Could you check a few things on this drawing? It's one solid part, dimensions in mm from its lowest x, y, z. A direction names the side the tool comes from. Coordinates: 2 decimals unless noted, no trailing zeros. Use one line per item in the form item = value. Start each with the question number.
(1) On a 3-axis mill with a long thin cutter (end or side, diameter ignored), from which of +Z, -Z, +X, -X, +Y, -Y can I reach the whole of each face in a straight line? I mean the marked faces 3 and 4. Say none if no direction works.
(2) Thinking about a two-plate mould opening in X: for the marked faces 1 and 2, which applies, +X half, -X half, draft (parallel to the pull), parting line (faces both ways), or undercut?
(3) Please list where these lines run through material, in increasing order: L1, parallel to Y at x = 20.5, z = 30; L2, parallel to Z at x = 31.5, y = 1.55; L3, parallel to X at y = 0.8, z = 53.5 (1 decimal).
(4) Will these pins go through, and if not, where does the flat tip stop? P1, Ø2, axis at x = 48, y = 2, coming from the -Z side; P2, Ø1, axis at y = 4, z = 37.5, coming from the +X side; P3, Ø3, axis at y = 1.5, z = 8, coming from the +X side (1 decimal).
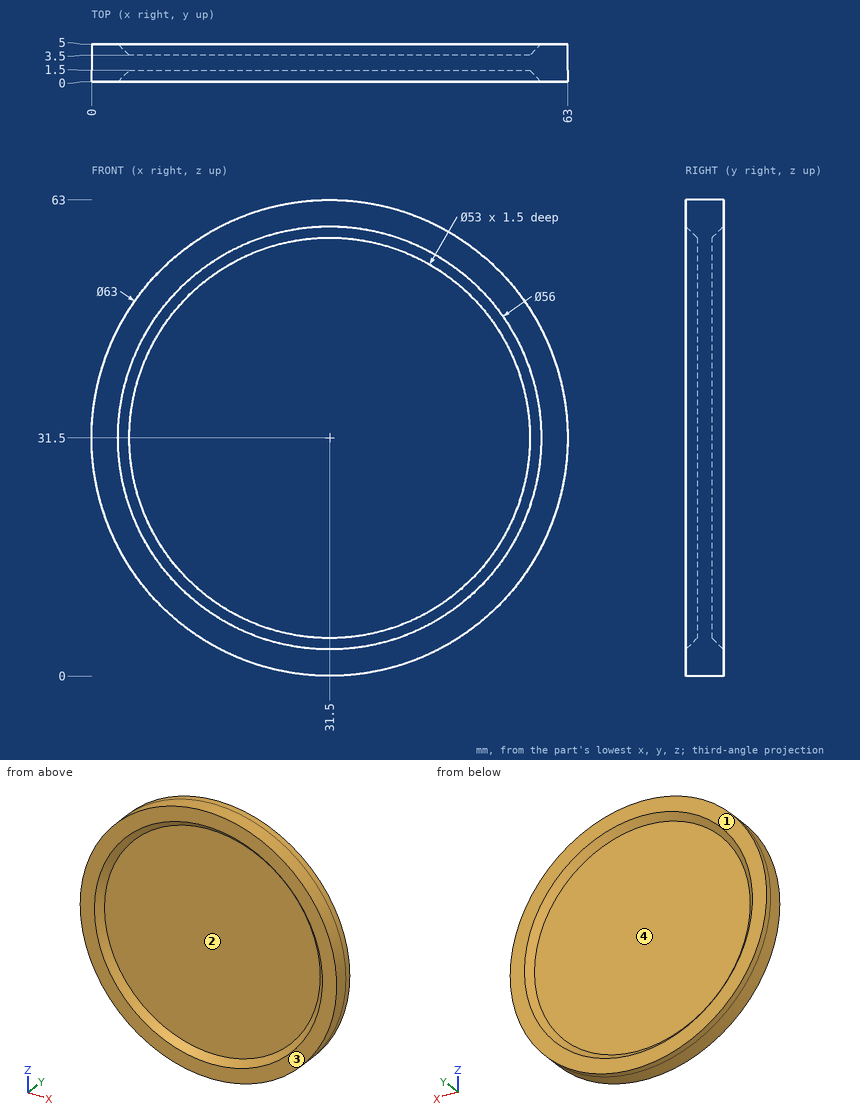
Answer:
q1.face_3 = +Z, -Z, +X, -X, -Y
q1.face_4 = +Y
q2.face_1 = draft
q2.face_2 = undercut
q3.L1 = 1.5 to 3.5
q3.L2 = 0 to 63
q3.L3 = 9 to 15.5, 47.5 to 54
q4.P1 = 4.08
q4.P2 = 62.52
q4.P3 = 54
